The model under review builds one solid part; all positions refer to its coordinate system, in mm. A direction names the side the tool comes from. Give positions to 0.01 mm unless a question says otherwise; leave off trailing zeros. Loops run counter-clockwise (first coordinate to the right, second up) from the corner with the lowest first, then second, coordinate; pieces in that order, holes last. Notation, with made-up numbers: M 25.5,56 L 32.5,56 A19 ccw 32.5,67 Z; hole C 5.25,83 d8. An arc over 180 degrees is marked long. Return JSON: item names as keys, results as strings.
```python
from build123d import *

# Parameters (mm, degrees)
STOCK_ROPE_START                        = -38.1
STOCK_ROPE_ROBOT_CHASSIS_MASTER_1_DEPTH = 76.2
CUT_EXTRUDE1_REACH                      = 392.081
SKETCH1_R                               = 15.24


# Read off the part's stored shape, not the designer's step: Stock-Rope Robot Chassis Master-1
with BuildPart() as part:
    # Stock-Rope Robot Chassis Master-1 outlin → Stock-Rope Robot Chassis Master-1 (new body)
    with BuildSketch(Plane.XY.offset(STOCK_ROPE_START)):
        with BuildLine():
            ThreePointArc((-127, -40.259), (-137.506899662, -35.906899662), (-141.859, -25.4))
            Line((-141.859, -25.4), (-141.859, 228.6))
            ThreePointArc((-141.859, 228.6), (-152.4, 239.141), (-162.941, 228.6))
            Line((-162.941, 228.6), (-161.925, 228.6))
            ThreePointArc((-161.925, 228.6), (-152.4, 238.125), (-142.875, 228.6))
            Line((-142.875, 228.6), (-142.875, -25.4))
            ThreePointArc((-142.875, -25.4), (-138.225320151, -36.625320151), (-127, -41.275))
            Line((-127, -41.275), (127, -41.275))
            ThreePointArc((127, -41.275), (138.225320151, -36.625320151), (142.875, -25.4))
            Line((142.875, -25.4), (142.875, 228.6))
            ThreePointArc((142.875, 228.6), (152.4, 238.125), (161.925, 228.6))
            Line((161.925, 228.6), (162.941, 228.6))
            ThreePointArc((162.941, 228.6), (152.4, 239.141), (141.859, 228.6))
            Line((141.859, 228.6), (141.859, -25.4))
            ThreePointArc((141.859, -25.4), (137.506899662, -35.906899662), (127, -40.259))
            Line((127, -40.259), (-127, -40.259))
        make_face()
    extrude(amount=STOCK_ROPE_ROBOT_CHASSIS_MASTER_1_DEPTH)

    # Sketch1 → Cut-Extrude1 (cut, up to next)
    with BuildSketch(Plane(origin=(142.875, 0, 0), x_dir=(0, 0, -1), z_dir=(1, 0, 0)), mode=Mode.PRIVATE) as cut_extrude1_sk1:
        with Locations(Location((0, 112.141, 0), (0, 0, 90))):
            Circle(SKETCH1_R)
    cut_extrude1_tool1 = extrude(cut_extrude1_sk1.sketch, amount=-CUT_EXTRUDE1_REACH, mode=Mode.PRIVATE) & part.part
    add(cut_extrude1_tool1.solids().sort_by_distance((142.875, 112.141, 0))[0], mode=Mode.SUBTRACT)


solid = part.part
```
1) Tool access review of faces 4 (the face through (142.875, 100, -17)), 5 (the face through (-141.859, 100, -1)), 6 (the face through (-152.609, 238.123, -0.533)): name each direction out of +Z, -Z, +X, -X, +Y, -Y from which nothing blocks a thin tool from reaching the whole face with its end or side.
From the geometry:
{"face 4": "+Z, -Z, +X, -Y", "face 5": "+Z, -Z, +Y", "face 6": "+Z, -Z, -Y"}
2) Consider section C-C on z = 32.5. Write out the cut boundary in (x, y) (3 decimals).
From the geometry:
{"outline": "M -162.941,228.6 L -161.925,228.6 A9.525 cw -142.875,228.6 L -142.875,-25.4 A15.875 ccw -127,-41.275 L 127,-41.275 A15.875 ccw 142.875,-25.4 L 142.875,228.6 A9.525 cw 161.925,228.6 L 162.941,228.6 A10.541 ccw 141.859,228.6 L 141.859,-25.4 A14.859 cw 127,-40.259 L -127,-40.259 A14.859 cw -141.859,-25.4 L -141.859,228.6 A10.541 ccw Z"}
3) Consider section B-B on z = 0. Write out the cut boundary in (x, y) (3 decimals), then the cut area to 3 significant figures.
From the geometry:
{"outline": "M -162.941,228.6 L -161.925,228.6 A9.525 cw -142.875,228.6 L -142.875,-25.4 A15.875 ccw -127,-41.275 L 127,-41.275 A15.875 ccw 142.875,-25.4 L 142.875,96.901 L 141.859,96.901 L 141.859,-25.4 A14.859 cw 127,-40.259 L -127,-40.259 A14.859 cw -141.859,-25.4 L -141.859,228.6 A10.541 ccw Z; M 141.859,127.381 L 142.875,127.381 L 142.875,228.6 A9.525 cw 161.925,228.6 L 162.941,228.6 A10.541 ccw 141.859,228.6 Z", "area": "856 mm²"}
4) The part is to be moulded in two halves that separate along Y. For faces 1 (the face through (-142.875, 103, -1)), 2 (the face through (142.374, 96.916, 0.67)), 3 (the face through (-138.35, -36.5, -0.53)), say which applies: released by +Y, released by -Y, zero draft, split by the parting line, or undercut.
From the geometry:
{"face 1": "zero draft", "face 2": "undercut", "face 3": "released by -Y"}
5) Wall thickness on L1, parallel to X at y = -4.5, z = -21.5 (3 decimals); L2, parallel to Y at x = 41, z = 14.5 (3 decimals); L3, parallel to X at y = -29.5, z = -32: over which ranges is each line inside the solid? List them lowest first. Write a range as from..to.
From the geometry:
{"L1": "-142.875..-141.859, 141.859..142.875", "L2": "-41.275..-40.259", "L3": "-142.34..-141.28, 141.28..142.34"}
6) Consider section D-D on x = 152.4. Write out the cut boundary in (y, z) (3 decimals), then the cut area to 3 significant figures.
From the geometry:
{"outline": "M 238.125,-38.1 L 239.141,-38.1 L 239.141,38.1 L 238.125,38.1 Z", "area": "77.4 mm²"}
7) Consider section A-A on y = 135. Write out the cut boundary in (x, z) (3 decimals).
From the geometry:
{"outline": "M -142.875,-38.1 L -141.859,-38.1 L -141.859,38.1 L -142.875,38.1 Z; M 141.859,-38.1 L 142.875,-38.1 L 142.875,38.1 L 141.859,38.1 Z"}
8) Insertion check: pin 1 (1 mm diameter, centred on x = 73, z = 0, fed in from +Y); pin 2 (23 mm diameter, centred on y = 71, z = 1, fed in from +X) (3 decimals); pin 3 (23 mm diameter, centred on y = 39.5, z = -12.5, fed in from -X) (3 decimals). Each pin has a flat end and moves straight along its axis. Give the tip position at first contact, or say it passes through.
From the geometry:
{"pin 1": "y = -40.26", "pin 2": "x = 142.875", "pin 3": "x = -142.875"}
